Job drawing, mm, ordinate dimensions from the low corner. One solid piece. Give positions to 0.01 mm unless a question says otherwise; leave off trailing zeros. Write each loop counter-clockwise with the first axis right and the second up, starting at its lowest first coordinate (ties: lowest second). Pieces come first, ordered by that corner, then holes. Notation, with made-up numbers: (-37.5, 46.25) -> (15.5, 46.25) arc R22 ccw to (15.5, 60.25) -> close; hole circle Ø2 at (20.25, 69.25). An arc over 180 degrees is marked (long way). One line per question, with ' | ' between items. Start each with the question number.
(1) Band-saw the part on B-B, the plane x = 136.5. Give the cut face in (y, z).
(2) Pin check, flat tip, straight feed: P1, Ø2, axis at y = 104.5, z = 33.5, coming from the +X side. Stop position of the tip, or through.
(3) Drill centre lines: probe 1 along X at (y, z) = (103, 47); probe 2 along X at (y, z) = (14, 45.5). Where is each one in solid material? Low to high. Write a range as from..to.
(4) Band-saw the part on A-A, the plane z = 48.5. Give the cut face in (x, y), and give its area (3 significant figures).
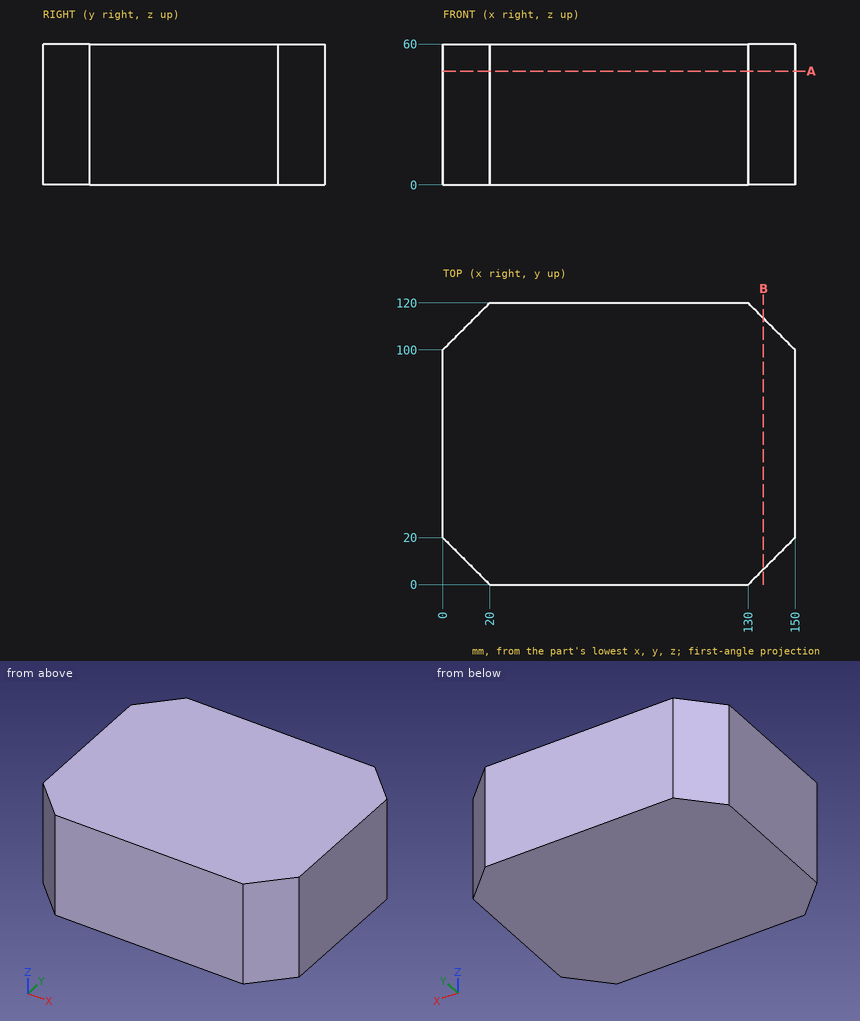
Results:
1) outline: (6.5, 0) -> (113.5, 0) -> (113.5, 60) -> (6.5, 60) -> close
2) P1: stops at x = 146.5
3) probe 1: x = 3..147 | probe 2: x = 6..144
4) outline: (0, 20) -> (20, 0) -> (130, 0) -> (150, 20) -> (150, 100) -> (130, 120) -> (20, 120) -> (0, 100) -> close | area: 17,200 mm²
